Could you check a few things on this model? Use its own coordinates, in mm. Face numbers are marked on the shaded views. A direction names the side the tool comes from. Coordinates: 2 decimals unless noted, no trailing zeros. Loops run counter-clockwise (first coordinate to the right, second up) from the corner with the lowest first, then second, coordinate; pieces in that order, holes last. Notation, with made-up numbers: (5, 44) - (36, 44) arc R14 cw to (36, 64) - close; hole circle Ø6 at (38.5, 38). An arc over 180 degrees is marked (long way). Use CSV: the item, a comma, the result in double quotes.
from build123d import *

# Parameters (mm, degrees)
CHAMFER1_SIZE = 4


with BuildPart() as part:
    # Sketch1 → Revolve1 (revolve)
    with BuildSketch(Plane(origin=(0, 0, 0), x_dir=(0, 0, -1), z_dir=(1, 0, 0))):
        Polygon((14, 12.175), (4.6, 12.175), (4.6, 16.175), (0, 16.175), (0, 12.175), (0, -12.825), (14, -12.825), (14, -7.825), (13, -7.825), (13, -6.825), (14, -6.825), align=None)
    revolve(axis=Axis((0, 12.175, 0), (0, -1, 0)))

    # Chamfer1
    chamfer1_edges = [part.edges().sort_by_distance(p)[0] for p in [
        (0, 12.175, 14),
    ]]
    chamfer(chamfer1_edges, length=CHAMFER1_SIZE)


solid = part.part
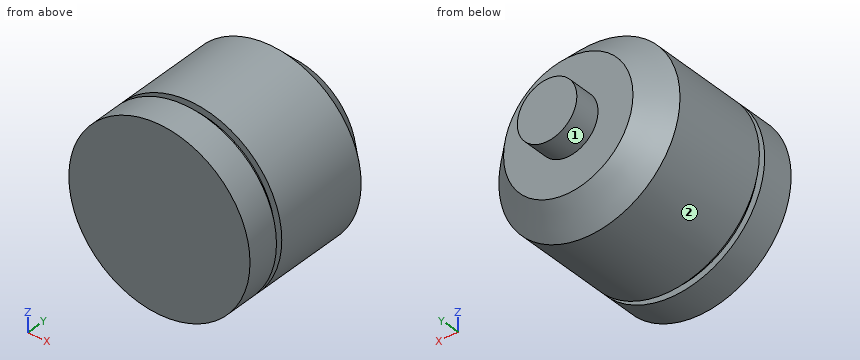
(1) Suppose I cut it at B-B (z = 0). Write out the boundary of the cut face in (x, y) (3 decimals), plus the area to 3 significant figures.
Computed:
outline,"(-14, -12.825) - (14, -12.825) - (14, -7.825) - (13, -7.825) - (13, -6.825) - (14, -6.825) - (14, 8.175) - (10, 12.175) - (4.6, 12.175) - (4.6, 16.175) - (-4.6, 16.175) - (-4.6, 12.175) - (-10, 12.175) - (-14, 8.175) - (-14, -6.825) - (-13, -6.825) - (-13, -7.825) - (-14, -7.825) - close"
area,"719 mm²"
(2) Suppose I cut it at A-A (x = 0). Write out the boundary of the cut face in (y, z) (3 decimals).
Computed:
outline,"(-12.825, -14) - (-7.825, -14) - (-7.825, -13) - (-6.825, -13) - (-6.825, -14) - (8.175, -14) - (12.175, -10) - (12.175, -4.6) - (16.175, -4.6) - (16.175, 4.6) - (12.175, 4.6) - (12.175, 10) - (8.175, 14) - (-6.825, 14) - (-6.825, 13) - (-7.825, 13) - (-7.825, 14) - (-12.825, 14) - close"
(3) Please list where these lines run through material, in increasing order: line 1 (Y direction, x = 6, z = 0) (3 decimals); line 2 (Y direction, x = 12.25, z = 5) (3 decimals); line 3 (X direction, y = -5.75, z = 8).
Computed:
line 1,"y = -12.825 to 12.175"
line 2,"y = -12.825 to -7.825, -6.825 to 8.944"
line 3,"x = -11.49 to 11.49"
(4) Suppose I cut it at C-C (y = 6.75). Write out the boundary of the cut face in (x, z).
Computed:
outline,"circle Ø28 at (0, 0)"
(5) Will these pins go through, and if not, where does the flat tip stop? pin 1 (8 mm diameter, centred on x = 8.5, z = 9, fed in from +Y) (3 decimals); pin 2 (2 mm diameter, centred on y = -3.5, z = -9, fed in from +X); pin 3 (2 mm diameter, centred on x = 6, y = -0.5, fed in from +Z).
Computed:
pin 1,"stops at y = 12.175"
pin 2,"stops at x = 11.49"
pin 3,"stops at z = 13.08"
(6) Which directions (+Z, -Z, +X, -X, +Y, -Y) give clear straight access to the entire face, cutting with the end or side of a thin tool? Please do the marked faces 1 and 2.
Computed:
face 1,"+Y"
face 2,"+Y, -Y"
